Read the model definition and answer for the solid it produces. Units are mm, in the model's axes. Face numbers are marked on the shaded views. A direction names the side the tool comes from. Give positions to 0.01 mm unless a question says otherwise; leave off trailing zeros. Order: outer loops, then holes, each group sorted by start corner. A loop starts at its lowest first (then second) coordinate and runs counter-clockwise, first axis right, second up. Notation, with made-up numbers: (77.25, 25) - (83.25, 25) arc R31 ccw to (83.25, 60) - close; hole circle Ø5 at (88.25, 81). An arc over 180 degrees is marked (long way). Use a Markdown table: item, result. Add a question column.
1. A cutting plane is placed at A-A on x = 0. Determine the outline of the cut face in (y, z), and give its area (3 significant figures).
2. Consider L1, parallel to Y at x = 0, z = 0.7; L2, parallel to Y at x = 0, z = 4.85; L3, parallel to Z at x = -10, y = 2. Determine where each line is inside the solid, lowest interval first.
3. For a pull along X with two mould halves and no side action, classify the marked faces 1, 2 and 3 as released by +X, released by -X, zero draft, split by the parting line, or undercut.
4. A cutting plane is placed at D-D on x = 7.5. Determine the outline of the cut face in (y, z).
5. Flat-ended cylindrical pins translate along their axes: P1, Ø4.5, axis at x = -0.5, y = -0.5, coming from the -Z side; P2, Ø4, axis at x = 2, y = 9.5, coming from the +Z side; P3, Ø3.5, axis at x = 0, y = 0, coming from the +Z side. Find the tip coordinate at first contact, or state that the pin passes through.
6. Which of the six approach directions +Z, -Z, +X, -X, +Y, -Y give full straight-line access (tool end or side, diameter ignored) to the marked faces 4 and 5?
7. A cutting plane is placed at C-C on z = 4.7. Determine the outline of the cut face in (x, y).
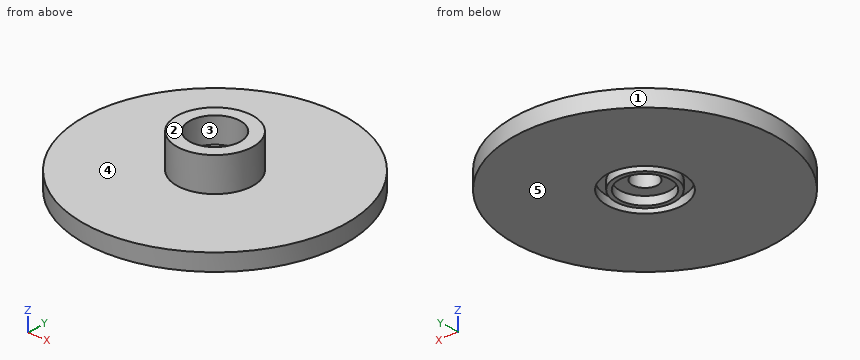
```python
from build123d import *

# Parameters (mm, degrees)
SCHIZZO1_R                   = 15.5
ESTRUSIONE_ESTRUSIONE1_DEPTH = 2
SCHIZZO2_R                   = 4.5
SCHIZZO2_R_2                 = 3
ESTRUSIONE_ESTRUSIONE2_DEPTH = 4
SCHIZZO3_R                   = 3
ESTRUSIONE_ESTRUSIONE3_DEPTH = 1
SCHIZZO4_R                   = 4.5
SCHIZZO4_R_2                 = 3.5
SCHIZZO4_R_3                 = 3
TAGLIO_ESTRUSIONE1_DEPTH     = 1
SCHIZZO5_R                   = 1.5
TAGLIO_ESTRUSIONE2_DEPTH     = 12


with BuildPart() as part:
    # Schizzo1 → Estrusione-Estrusione1 (new body)
    with BuildSketch(Plane.XY):
        Circle(SCHIZZO1_R)
    extrude(amount=ESTRUSIONE_ESTRUSIONE1_DEPTH)

    # Schizzo2 → Estrusione-Estrusione2 (add)
    with BuildSketch(Plane.XY.offset(2)):
        Circle(SCHIZZO2_R)
        Circle(SCHIZZO2_R_2, mode=Mode.SUBTRACT)
    extrude(amount=ESTRUSIONE_ESTRUSIONE2_DEPTH)

    # Schizzo3 → Estrusione-Estrusione3 (add)
    with BuildSketch(Plane.XY.offset(2)):
        Circle(SCHIZZO3_R)
    extrude(amount=ESTRUSIONE_ESTRUSIONE3_DEPTH)

    # Schizzo4 → Taglio-Estrusione1 (cut)
    with BuildSketch(Plane(origin=(0, 0, 0), x_dir=(-1, 0, 0), z_dir=(0, 0, -1))):
        with Locations(Location((0, 0, 0), (0, 0, 180))):
            Circle(SCHIZZO4_R)
        Circle(SCHIZZO4_R_2, mode=Mode.SUBTRACT)
        with Locations(Location((0, 0, 0), (0, 0, 180))):
            Circle(SCHIZZO4_R_3)
    extrude(amount=-TAGLIO_ESTRUSIONE1_DEPTH, mode=Mode.SUBTRACT)

    # Schizzo5 → Taglio-Estrusione2 (cut)
    with BuildSketch(Plane(origin=(0, 0, 1), x_dir=(-1, 0, 0), z_dir=(0, 0, -1))):
        Circle(SCHIZZO5_R)
    extrude(amount=-TAGLIO_ESTRUSIONE2_DEPTH, mode=Mode.SUBTRACT)


solid = part.part
```
Output values:
| question | item | result |
|---|---|---|
| 1 | outline | (-15.5, 0) - (-4.5, 0) - (-4.5, 1) - (-3.5, 1) - (-3.5, 0) - (-3, 0) - (-3, 1) - (-1.5, 1) - (-1.5, 3) - (-3, 3) - (-3, 6) - (-4.5, 6) - (-4.5, 2) - (-15.5, 2) - close; (1.5, 1) - (3, 1) - (3, 0) - (3.5, 0) - (3.5, 1) - (4.5, 1) - (4.5, 0) - (15.5, 0) - (15.5, 2) - (4.5, 2) - (4.5, 6) - (3, 6) - (3, 3) - (1.5, 3) - close |
| 1 | area | 66.0 mm² |
| 2 | L1 | -15.5 to -4.5, -3.5 to -3, 3 to 3.5, 4.5 to 15.5 |
| 2 | L2 | -4.5 to -3, 3 to 4.5 |
| 2 | L3 | 0 to 2 |
| 3 | face 1 | split by the parting line |
| 3 | face 2 | zero draft |
| 3 | face 3 | undercut |
| 4 | outline | (-13.56, 0) - (13.56, 0) - (13.56, 2) - (-13.56, 2) - close |
| 5 | P1 | z = 1 |
| 5 | P2 | z = 2 |
| 5 | P3 | z = 3 |
| 6 | face 4 | +Z |
| 6 | face 5 | -Z, +X, -X, +Y, -Y |
| 7 | outline | circle Ø9 at (0, 0); hole circle Ø6 at (0, 0) |
